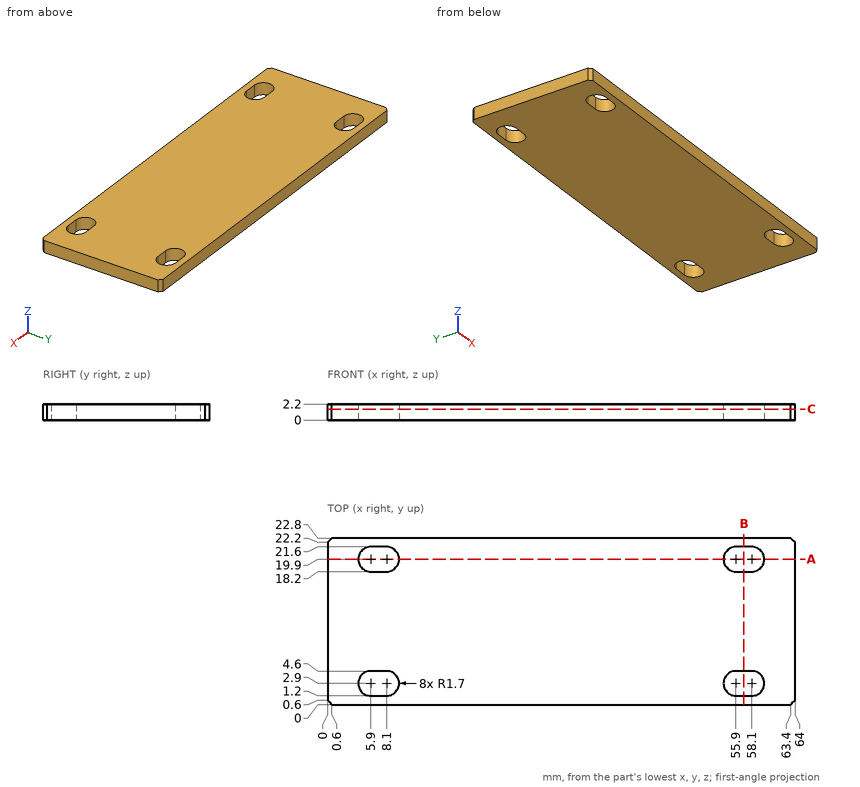
The figure shows three views and two pictorial views of one solid part (mm, origin at its lowest corner). Answer the questions. Coordinates: 2 decimals unless noted, no trailing zeros. Loops run counter-clockwise (first coordinate to the right, second up) from the corner with the lowest first, then second, coordinate; pieces in that order, holes last. Notation, with made-up numbers: (-7.5, -12) - (16.5, -12) arc R28 ccw to (16.5, 9) - close; hole circle Ø1 at (-9.5, 77.25). An arc over 180 degrees is marked (long way). Write item = value, one per line.
1) Section B-B (x = 57) is taken. Determine the outline of the cut face in (y, z).
Responses:
outline = (0, 0) - (1.2, 0) - (1.2, 2.2) - (0, 2.2) - close; (4.6, 0) - (18.2, 0) - (18.2, 2.2) - (4.6, 2.2) - close; (21.6, 0) - (22.8, 0) - (22.8, 2.2) - (21.6, 2.2) - close
2) This flat-tipped pin is pushed along its axis until it touches: P1, Ø0.7, axis at x = 6.5, z = 0.5, coming from the -Y side. Where does it stop, or does it pass through?
Responses:
P1 = 0
3) Section A-A (y = 19.9) is taken. Determine the outline of the cut face in (x, z), plus the area to 3 significant figures.
Responses:
outline = (0, 0) - (4.2, 0) - (4.2, 2.2) - (0, 2.2) - close; (9.8, 0) - (54.2, 0) - (54.2, 2.2) - (9.8, 2.2) - close; (59.8, 0) - (64, 0) - (64, 2.2) - (59.8, 2.2) - close
area = 116 mm^2
4) Find the intervals of material crossed by line 1 along Y through (x, z) = (6, 0.3); line 2 along X through (y, z) = (3, 1); line 3 along Y through (x, z) = (5, 1.1), in increasing order.
Responses:
line_1 = 0 to 1.2, 4.6 to 18.2, 21.6 to 22.8
line_2 = 0 to 4.2, 9.8 to 54.2, 59.8 to 64
line_3 = 0 to 1.46, 4.34 to 18.46, 21.34 to 22.8
5) Section C-C (z = 1.5) is taken. Determine the outline of the cut face in (x, y), plus the area to 3 significant figures.
Responses:
outline = (0, 0.6) - (0.6, 0) - (63.4, 0) - (64, 0.6) - (64, 22.2) - (63.4, 22.8) - (0.6, 22.8) - (0, 22.2) - close; hole (5.9, 1.2) - (8.1, 1.2) arc R1.7 ccw to (8.1, 4.6) - (5.9, 4.6) arc R1.7 ccw to start; hole (5.9, 18.2) - (8.1, 18.2) arc R1.7 ccw to (8.1, 21.6) - (5.9, 21.6) arc R1.7 ccw to start; hole (55.9, 1.2) - (58.1, 1.2) arc R1.7 ccw to (58.1, 4.6) - (55.9, 4.6) arc R1.7 ccw to start; hole (55.9, 18.2) - (58.1, 18.2) arc R1.7 ccw to (58.1, 21.6) - (55.9, 21.6) arc R1.7 ccw to start
area = 1,390 mm^2
